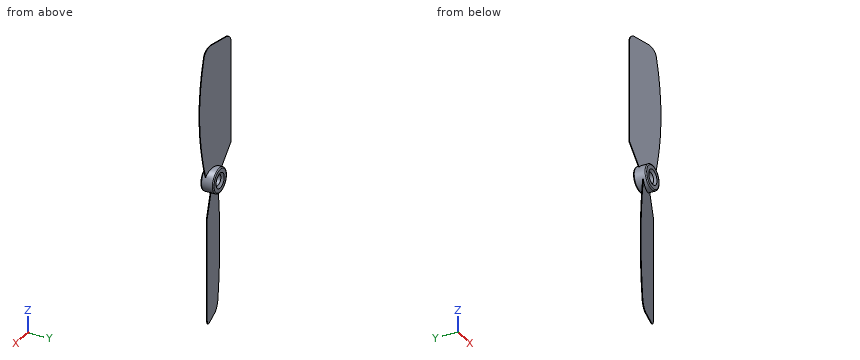
```python
from build123d import *

# Parameters (mm, degrees)
SKETCH1_R           = 5.75
BOSS_EXTRUDE1_DEPTH = 3
BOSS_EXTRUDE3_DEPTH = 0.15
CIRPATTERN1_COUNT   = 2
SKETCH5_R           = 2.5
CUT_EXTRUDE1_DEPTH  = 65.596843827
FILLET1_R           = 0.5
FILLET2_SIZE        = 1


with BuildPart() as part:
    # Sketch1 → Boss-Extrude1 (new, symmetric)
    with BuildSketch(Plane(origin=(0, 0, 0), x_dir=(1, 0, 0), z_dir=(0, 1, 0))):
        with Locations(Location((0, 0, 0), (0, 0, 270))):
            Circle(SKETCH1_R)
    extrude(amount=BOSS_EXTRUDE1_DEPTH, both=True)

    # Sketch3 → Boss-Extrude3 (add, symmetric)
    with BuildSketch(Plane(origin=(0, 0, 0), x_dir=(0.9743700647852351, -0.22495105434386542, 0), z_dir=(-0.22495105434386542, -0.9743700647852351, 0))):
        with BuildLine():
            ThreePointArc((-4.185847137, 2.859510833), (0.450269951, 5.535994412), (5.086387038, 2.859510833))
            add(Edge.make_bspline(
                [(5.086387038, 2.859510833), (12.031976461, 30.617463191), (6.126015088, 59.154329089)],
                knots=[0, 0, 0, 1, 1, 1], degree=2))
            ThreePointArc((6.126015088, 59.154329089), (4.465099784, 62.259763653), (1.16901464, 63.5))
            Line((1.16901464, 63.5), (-7.456899563, 63.5))
            ThreePointArc((-7.456899563, 63.5), (-9.578219907, 62.621320344), (-10.456899563, 60.5))
            Line((-10.456899563, 60.5), (-10.456899563, 12.886138045))
            Line((-10.456899563, 12.886138045), (-4.185847137, 2.859510833))
        make_face()
    boss_extrude3 = extrude(amount=BOSS_EXTRUDE3_DEPTH, both=True)

    # CirPattern1: Boss-Extrude3 ×2 about axis
    cirpattern1_axis = Axis((0, 3, 0), (0, -1, 0))
    for i in range(1, CIRPATTERN1_COUNT):
        add(boss_extrude3.rotate(cirpattern1_axis, i * 360 / CIRPATTERN1_COUNT))

    # Sketch5 → Cut-Extrude1 (cut, through all)
    with BuildSketch(Plane(origin=(0, 3, 0), x_dir=(1, 0, 0), z_dir=(0, 1, 0))):
        with Locations(Location((0, 0, 0), (0, 0, 270))):
            Circle(SKETCH5_R)
    extrude(amount=-CUT_EXTRUDE1_DEPTH, mode=Mode.SUBTRACT)

    # Fillet1
    fillet1_edges = [part.edges().sort_by_distance(p)[0] for p in [
        (0, -3, -5.75),
        (0, 3, -5.75),
    ]]
    fillet(fillet1_edges, radius=FILLET1_R)

    # Fillet2
    fillet2_edges = [part.edges().sort_by_distance(p)[0] for p in [
        (0, -3, -2.5),
        (0, 3, -2.5),
    ]]
    chamfer(fillet2_edges, length=FILLET2_SIZE)


solid = part.part
```
CAD build for the part. Positions are in the model's coordinates, mm. Coordinates: 2 decimals unless noted, no trailing zeros. Order: outer loops, then holes, each group sorted by start corner. A loop starts at its lowest first (then second) coordinate and runs counter-clockwise, first axis right, second up. Notation, with made-up numbers: (-14, 32.25) - (15, 32.25) arc R17 cw to (15, 41.25) - close; hole circle Ø7 at (-29, 30). An arc over 180 degrees is marked (long way). Use a Markdown table: item, result. Add a question column.
(1) Saw through at B-B (z = 0). Give the cut face in (x, y).
(2) Flat gauge pins, fed straight in: pin 1 (4 mm diameter, centred on x = -7, z = -23.5, fed in from +Y); pin 2 (4 mm diameter, centred on x = -7.5, z = 5, fed in from +Y); pin 3 (3 mm diameter, centred on x = -5.5, z = -39.5, fed in from +Y). Where does each tip first touch, or does it go through?
(3) Drill centre lines: line 1 along X through (y, z) = (-0.6, 0); line 2 along Y through (x, z) = (3.5, 4); line 3 along Y through (x, z) = (4.5, -26). Where is each one in solid material? Low to high. Write a range as [from, to].
(4) Saw through at A-A (x = 0). Give the cut face in (y, z), then the cut area to 3 significant figures.
Solved:
| question | item | result |
|---|---|---|
| 1 | outline | (-5.75, -2.5) arc R0.5 ccw to (-5.25, -3) - (-3.5, -3) - (-2.5, -2) - (-2.5, 2) - (-3.5, 3) - (-5.25, 3) arc R0.5 ccw to (-5.75, 2.5) - close; (2.5, -2) - (3.5, -3) - (5.25, -3) arc R0.5 ccw to (5.75, -2.5) - (5.75, 2.5) arc R0.5 ccw to (5.25, 3) - (3.5, 3) - (2.5, 2) - close |
| 2 | pin 1 | stops at y = -1 |
| 2 | pin 2 | stops at y = 1.62 |
| 2 | pin 3 | stops at y = -0.77 |
| 3 | line 1 | x = [-5.75, -2.5], [2.5, 5.75] |
| 3 | line 2 | y = [-3, 3] |
| 3 | line 3 | y = [0.88, 1.19] |
| 4 | outline | (-3, -5.25) arc R0.5 ccw to (-2.5, -5.75) - (-0.15, -5.75) - (-0.15, -63.5) - (0.15, -63.5) - (0.15, -5.75) - (2.5, -5.75) arc R0.5 ccw to (3, -5.25) - (3, -3.5) - (2, -2.5) - (-2, -2.5) - (-3, -3.5) - close; (-3, 3.5) - (-2, 2.5) - (2, 2.5) - (3, 3.5) - (3, 5.25) arc R0.5 ccw to (2.5, 5.75) - (0.15, 5.75) - (0.15, 63.5) - (-0.15, 63.5) - (-0.15, 5.75) - (-2.5, 5.75) arc R0.5 ccw to (-3, 5.25) - close |
| 4 | area | 72.3 mm² |
